Verification items for the finished model (mm, model axes). A direction names the side the tool comes from. Give positions to 0.01 mm unless a question says otherwise; leave off trailing zeros. Order: outer loops, then holes, each group sorted by start corner. A loop starts at its lowest first (then second) coordinate and runs counter-clockwise, first axis right, second up. Notation, with made-up numbers: (45, 0.25) - (84, 0.25) arc R11 cw to (84, 9.25) - close; hole circle Ø4 at (24, 49.25). An arc over 180 degrees is marked (long way). Answer as a JSON object with one key per item and string values. Group by question number.
(1) Mould release check, pull along Y, two halves, no side actions. Record for faces 1 (the face through (20, 20, 0)), 2 (the face through (-19.72, 15.12, 16.47)), 3 (the face through (-19.98, -0.88, 13.66)), 4 (the face through (-28.943, 19.476, 4.556)): +Y half, -Y half, draft (parallel to the pull), parting line (faces both ways), or undercut.
(2) Depth check by flat-ended pin: pin 1 Ø3 at (x, y) = (-19, -24) entering from -Z; pin 2 Ø5 at (x, z) = (-3, 2.5) entering from +Y; pin 3 Ø21 at (x, y) = (9.5, -1) entering from +Z. Enter the tip coordinate at first touch or a pass-through.
(3) Access from +Z, -Z, +X, -X, +Y, -Y to the whole of each face (thin tool, end or side, straight path). Record for faces 5 (the face through (-19, 8, 10.75)), 6 (the face through (-0.705, 33.827, 4.556)), 7 (the face through (-19.98, -0.88, 2.17)), 8 (the face through (-16.35, 12.53, -13.17)).
(4) Section check B-B (z = -4.5). Record the boundary of the cut face in (x, y), then the cut area to 3 significant figures.
(5) Thickness scan on line 1 (Y direction, x = -31, z = 3); line 2 (Y direction, x = 0, z = 16.65); line 3 (X direction, y = 18, z = 7). Record the ranges inside material, lowest first.
(6) Section check A-A (x = 0). Count the separate pieces of the cut face and the enclosed holes in it, then the cut area to 3 significant figures.
```python
from build123d import *

# Parameters (mm, degrees)
CROQUIS2_R            = 3.25
CORTAR_EXTRUIR1_DEPTH = 71.334930867
CHAFL_N1_SIZE         = 0.5


with BuildPart() as part:
    # Croquis1 → Revolución1 (revolve)
    with BuildSketch(Plane(origin=(0, 0, 0), x_dir=(0, 0, -1), z_dir=(1, 0, 0)), mode=Mode.PRIVATE) as revoluci_n1_sk:
        with BuildLine():
            Line((-9, 26.216025404), (-9, 45.5))
            Line((-9, 45.5), (-8, 46.5))
            Line((-8, 46.5), (-1, 46.5))
            Line((-1, 46.5), (0, 45.5))
            Line((0, 45.5), (0, 26))
            ThreePointArc((0, 26), (0.3, 25.7), (0.6, 26))
            Line((0.6, 26), (15.45, 26))
            Line((15.45, 26), (15.95, 25.5))
            Line((15.95, 25.5), (15.95, 21.1))
            Line((15.95, 21.1), (15.45, 20.6))
            Line((15.45, 20.6), (10.95, 20.6))
            Line((10.95, 20.6), (10.95, 18.7))
            Line((10.95, 18.7), (10.75, 18.5))
            Line((10.75, 18.5), (7.65, 18.5))
            Line((7.65, 18.5), (7.45, 18.7))
            Line((7.45, 18.7), (7.45, 19.2))
            ThreePointArc((7.45, 19.2), (7.215685425, 19.765685425), (6.65, 20))
            Line((6.65, 20), (-10.75, 20))
            Line((-10.75, 20), (-10.75, 21.25))
            Line((-10.75, 21.25), (-13.05, 21.25))
            Line((-13.05, 21.25), (-13.05, 20))
            Line((-13.05, 20), (-14.25, 20))
            Line((-14.25, 20), (-14.25, 20.6))
            Line((-14.25, 20.6), (-18.75, 20.6))
            Line((-18.75, 20.6), (-19.25, 21.1))
            Line((-19.25, 21.1), (-19.25, 24.35))
            Line((-19.25, 24.35), (-18.75, 24.85))
            Line((-18.75, 24.85), (-14.25, 24.85))
            Line((-14.25, 24.85), (-13.75, 25.35))
            Line((-13.75, 25.35), (-9.5, 25.35))
            ThreePointArc((-9.5, 25.35), (-9.133974596, 25.716025404), (-9, 26.216025404))
        make_face()
    revolve(revoluci_n1_sk.sketch.rotate(Axis((0, 0, 23.302641181), (0, 0, -1)), 90), axis=Axis((0, 0, 23.302641181), (0, 0, -1)))

    # Croquis2 → Cortar-Extruir1 (cut, through all)
    with BuildSketch(Plane.XY.offset(9)):
        with Locations((0, 37)):
            Circle(CROQUIS2_R)
        with Locations((32.04293994, 18.5)):
            Circle(CROQUIS2_R)
        with Locations((32.04293994, -18.5)):
            Circle(CROQUIS2_R)
        with Locations((0, -37)):
            Circle(CROQUIS2_R)
        with Locations((-32.04293994, -18.5)):
            Circle(CROQUIS2_R)
        with Locations((-32.04293994, 18.5)):
            Circle(CROQUIS2_R)
    extrude(amount=-CORTAR_EXTRUIR1_DEPTH, mode=Mode.SUBTRACT)

    # Chaflán1
    chafl_n1_edges = [part.edges().sort_by_distance(p)[0] for p in [
        (-3.25, 37, 0),
        (-3.25, 37, 9),
        (-35.29293994, 18.5, 0),
        (-35.29293994, 18.5, 9),
        (-35.29293994, -18.5, 0),
        (-35.29293994, -18.5, 9),
        (-3.25, -37, 0),
        (-3.25, -37, 9),
        (28.79293994, -18.5, 0),
        (28.79293994, -18.5, 9),
        (28.79293994, 18.5, 0),
        (28.79293994, 18.5, 9),
    ]]
    chamfer(chafl_n1_edges, length=CHAFL_N1_SIZE)


solid = part.part
```
Solutions:
{
 "1": {"face 1": "draft", "face 2": "parting line", "face 3": "undercut", "face 4": "undercut"},
 "2": {"pin 1": "stops at z = 0", "pin 2": "stops at y = 46.5", "pin 3": "stops at z = 14.25"},
 "3": {"face 5": "none", "face 6": "+Z, -Z", "face 7": "+Z", "face 8": "-Z"},
 "4": {"outline": "circle Ø52 at (0, 0); hole circle Ø40 at (0, 0)", "area": "867 mm2"},
 "5": {"line 1": "y = -34.66 to -21.58, -15.42 to 15.42, 21.58 to 34.66", "line 2": "y = -24.85 to -20.6, 20.6 to 24.85", "line 3": "x = -42.87 to -35.25, -28.83 to -8.72, 8.72 to 28.83, 35.25 to 42.87"},
 "6": {"separate pieces": "4", "enclosed holes": "0", "area": "645 mm2"}
}
